Design review of the part built by this model. Coordinates are the model's own, in mm. A direction names the side the tool comes from. Coordinates: 2 decimals unless noted, no trailing zeros. Loops run counter-clockwise (first coordinate to the right, second up) from the corner with the lowest first, then second, coordinate; pieces in that order, holes last. Notation, with made-up numbers: (33.5, 78.5) -> (82.5, 78.5) arc R35 ccw to (82.5, 110.5) -> close; hole circle Ø10 at (32, -40). An arc over 180 degrees is marked (long way). Use a Markdown table: item, result. Add a question column.
Q1. Take a section at C-C on y = 25. Count the separate pieces of the cut face and the enclosed holes in it, plus the area to 3 significant figures.
Q2. Clearance check with flat-ended pins moving along their axes: pin 1 Ø1.2 at (x, z) = (16.5, 3.5) entering from -Y; pin 2 Ø1 at (y, z) = (5.5, 2) entering from -X; pin 3 Ø1.5 at (y, z) = (9, 5.5) entering from -X; pin 4 Ø1.2 at (x, z) = (-15.91, 4) entering from +Y. State where each tip first meets the part, or that it passes through.
Q3. For faces 5 (the face through (13.315, -1.506, 1.87)), 6 (the face through (11.89, 16.42, 6.86)), 7 (the face through (16, -2.52, 5)), list the 3-axis set-ups (+Z, -Z, +X, -X, +Y, -Y) from which the entire face can be reached by the end or side of a thin tool; tool diameter is ignored.
Q4. Draft analysis for pull direction Y (two halves, no side actions). For faces 1 (the face through (-14, -1.92, 4)), 2 (the face through (3, 16, 8)), 3 (the face through (11.89, 16.42, 1.14)), 4 (the face through (16, 9.48, 4)), state which applies: pulls with the +Y half, pulls with the -Y half, needs draft (parallel to the pull), parting line crosses it, or undercut.
Q5. Take a section at D-D on x = 6.5. Write out the cut boundary in (y, z), plus the area to 3 significant figures.
Q6. For probe 1 along Y at (x, z) = (14.5, 6.5); probe 2 along Y at (x, z) = (-14.5, 4.5); probe 3 along X at (y, z) = (12, 4.25), list the stretches that pass through material, from the lowest coordinate up.
from build123d import *

# Parameters (mm, degrees)
F1_DEPTH = 8
F2_R     = 3.99999
F3_R     = 1
F4_DEPTH = 60
F6_R     = 3.99999
F5_R     = 3.5
F7_DEPTH = 2
F8_R     = 0.75
F9_DEPTH = 12


# Not quite as in the source:
# - a fillet or chamfer is up to 0.001 mm smaller than in the source, because OpenCascade refuses the exact size


with BuildPart() as f1:
    # F0 (on Top) → F1 (new body)
    with BuildSketch(Plane.XY):
        Polygon((-19.9077894302, -1.920078908), (-19.9077894302, -12.520078908), (-1.9077894302, -12.520078908), (-1.9077894302, -0.520078908), (27.0922105698, -0.520078908), (27.0922105698, 10.079921092), (13.0922105698, 10.079921092), (13.0922105698, 22.579921092), (27.0922105698, 22.579921092), (27.0922105698, 33.179921092), (-19.9077894302, 33.179921092), (-19.9077894302, 22.579921092), (-9.9077894302, 22.579921092), (-9.9077894302, -1.920078908), align=None)
    extrude(amount=F1_DEPTH)

    # F2 (radius 4 in the source; OpenCascade refuses exactly that, so slightly less here)
    f2_edges = [f1.edges().sort_by_distance(p)[0] for p in [
        (-19.907789, -7.220079, 8),
        (-19.907789, -7.220079, 0),
        (-1.907789, -6.520079, 8),
        (-1.907789, -6.520079, 0),
        (27.092211, 4.779921, 8),
        (27.092211, 4.779921, 0),
        (27.092211, 27.879921, 8),
        (27.092211, 27.879921, 0),
        (-19.907789, 27.879921, 8),
        (-19.907789, 27.879921, 0),
    ]]
    fillet(f2_edges, radius=F2_R)

    # F3 (on face) → F4 (cut)
    with BuildSketch(Plane(origin=(0, 33.179921092, 0), x_dir=(-1, 0, 0), z_dir=(0, 1, 0))):
        with Locations((-23.0922105698, 4)):
            Circle(F3_R)
        with Locations((15.9077894302, 4)):
            Circle(F3_R)
    extrude(amount=-F4_DEPTH, mode=Mode.SUBTRACT)

    # F6 (radius 4 in the source; OpenCascade refuses exactly that, so slightly less here)
    f6_edges = [f1.edges().sort_by_distance(p)[0] for p in [
        (-9.907789, 10.329921, 8),
        (-9.907789, 10.329921, 0),
        (13.092211, 16.329921, 8),
        (13.092211, 16.329921, 0),
    ]]
    fillet(f6_edges, radius=F6_R)

    # F5 (on face) → F7 (join)
    with BuildSketch(Plane.XZ.offset(0.520078908)):
        with Locations((16.0922105698, 4)):
            Circle(F5_R)
    extrude(amount=F7_DEPTH)

    # F8 (on face) → F9 (cut)
    with BuildSketch(Plane.XZ.offset(2.520078908)):
        with Locations((16.0922105698, 4)):
            Circle(F8_R)
    extrude(amount=-F9_DEPTH, mode=Mode.SUBTRACT)


solid = f1.part
Answer list:
| question | item | result |
|---|---|---|
| 1 | separate pieces | 1 |
| 1 | enclosed holes | 2 |
| 1 | area | 356 mm² |
| 2 | pin 1 | y = -2.52 |
| 2 | pin 2 | x = -9.62 |
| 2 | pin 3 | x = -9.84 |
| 2 | pin 4 | through |
| 3 | face 5 | -Y |
| 3 | face 6 | +Z, +X |
| 3 | face 7 | +Z, -Z, +X, -Y |
| 4 | face 1 | undercut |
| 4 | face 2 | needs draft |
| 4 | face 3 | undercut |
| 4 | face 4 | pulls with the -Y half |
| 5 | outline | (-0.52, 0) -> (33.18, 0) -> (33.18, 8) -> (-0.52, 8) -> close |
| 5 | area | 270 mm² |
| 6 | probe 1 | -2.52 to 10.08, 22.58 to 33.18 |
| 6 | probe 2 | -12.52 to -1.92, 22.58 to 33.18 |
| 6 | probe 3 | -9.9 to 13.08 |
